Geometry: final body of the model. Coordinates: model frame, mm. A direction names the side the tool comes from. Round coordinates to 2 decimals unless told otherwise and drop trailing zeros. Loops run counter-clockwise (first coordinate to the right, second up) from the corner with the lowest first, then second, coordinate; pieces in that order, holes last. Notation, with made-up numbers: (85.5, 4) - (100.5, 4) arc R18 ccw to (100.5, 33) - close; hole circle Ø2 at (-11.75, -17.75). An arc over 180 degrees is marked (long way). Return JSON: item names as keys, results as strings. Group by question number.
1. Section D-D on y = -36.5. Return loops of the section in (x, z) (3 decimals).
2. Set-up query: faces 5 (the face through (4, -6.858, 33)), 6 (the face through (45.8, -0.2, 38.1)), 7 (the face through (37.434, -9.855, 55.828)), 8 (the face through (41.275, 0, 4)). Return all of +Z, -Z, +X, -X, +Y, -Y with unobstructed straight access to the full face (end or side cutting, diameter ignored); none if empty.
3. Section A-A on y = -24.5. Return loops of the section in (x, z) (3 decimals).
4. Section B-B on z = 5. Return loops of the section in (x, y) (3 decimals), and give its area (3 significant figures).
5. Draft query along X for faces 1 (the face through (60, 0, 42.875)), 2 (the face through (56, 14.478, 45)), 3 (the face through (139.48, -0.97, 52.19)), 4 (the face through (61.811, 0, 41)). Return one class per face: +X half, -X half, draft (parallel to the pull), parting line (faces both ways), or undercut.
6. Section C-C on x = 111. Return loops of the section in (y, z) (3 decimals), and give its area (3 significant figures).
7. Material intervals for probe 1 along Z at (x, y) = (81.5, -8.5) (3 decimals); probe 2 along Y at (x, z) = (24, 42); probe 3 along Z at (x, y) = (38, -25.5) (3 decimals), sorted ascending.
8. First-contact query: pin 1 Ø2.5 at (y, z) = (-1.5, 40) entering from -X; pin 2 Ø16 at (x, y) = (108, -3.5) entering from -Z; pin 3 Ø5 at (y, z) = (-2.5, 65.5) entering from -X; pin 4 Ø8 at (x, y) = (61, -5.5) entering from +Z (3 decimals). Flat tips, straight axial feed; report the tip coordinate or a pass-through.
from build123d import *

# Parameters (mm, degrees)
F1_DEPTH = 41.91
F0_W     = 23.9135493911
F0_H     = 19.0500000095
F0_H_2   = 4.7497999905
F0_H_3   = 4.7752
F2_DEPTH = 14.478
F3_DEPTH = 6.858
F5_R     = 15.24
F6_SIZE  = 5.08


with BuildPart() as f1:
    # F0 (on Front) → F1 (new body, symmetric)
    with BuildSketch(Plane.XZ):
        Polygon((22.2249999905, 9.525), (-41.275, 9.525), (-41.275, -9.525), (41.275, -9.525), (41.275, 9.525), align=None)
    extrude(amount=F1_DEPTH, both=True)

    # F0 (on Front) → F2 (join, symmetric)
    with BuildSketch(Plane.XZ):
        with Locations((73.7682253044, 52.4002000047)):
            Rectangle(F0_W, F0_H)
        Polygon((85.725, 66.675), (85.725, 61.9252000095), (85.725, 42.8752), (85.725, 38.1), (112.6114506089, 38.1), (112.6114506089, 66.675), align=None)
        with Locations((73.7682253044, 64.3001000047)):
            Rectangle(F0_W, F0_H_2)
        with Locations((73.7682253044, 40.4876)):
            Rectangle(F0_W, F0_H_3)
        with BuildLine():
            Line((22.2249999905, 27.0002), (22.2249999905, 9.525))
            Line((22.2249999905, 9.525), (41.275, 9.525))
            Line((41.275, 9.525), (41.275, 27.0002))
            ThreePointArc((41.275, 27.0002), (45.9246798487, 38.2255201513), (57.15, 42.8752))
            Line((57.15, 42.8752), (61.8114506089, 42.8752))
            Line((61.8114506089, 42.8752), (61.8114506089, 61.9252000095))
            Line((61.8114506089, 61.9252000095), (57.15, 61.9252000095))
            ThreePointArc((57.15, 61.9252000095), (52.4471910202, 61.6071243557), (47.8300426869, 60.6586910735))
            ThreePointArc((47.8300426869, 60.6586910735), (29.3538209918, 48.1456027677), (22.2249999905, 27.0002))
        make_face()
    extrude(amount=F2_DEPTH, both=True)

    # F0 (on Front) → F3 (join, symmetric)
    with BuildSketch(Plane.XZ):
        with BuildLine():
            add(Edge.make_bspline(
                [(-41.275, 9.525), (-40.409822017, 35.7104353607), (5.303404294, 69.4405809045), (47.8300426869, 60.6586910735)],
                knots=[0, 0, 0, 0, 102.734429453, 102.734429453, 102.734429453, 102.734429453], degree=3))
            Line((-41.275, 9.525), (22.2249999905, 9.525))
            Line((22.2249999905, 9.525), (22.2249999905, 27.0002))
            ThreePointArc((22.2249999905, 27.0002), (29.3538209918, 48.1456027677), (47.8300426869, 60.6586910735))
        make_face()
    extrude(amount=F3_DEPTH, both=True)

    # F0 (on Front) → F4 (revolve)
    with BuildSketch(Plane.XZ):
        Polygon((85.725, 66.675), (85.725, 61.9252000095), (85.725, 42.8752), (85.725, 38.1), (112.6114506089, 38.1), (112.6114506089, 66.675), align=None)
    revolve(axis=Axis((112.6114506089, 0, 52.3875), (0, 0, 1)))

    # F5
    f5_edges = [f1.edges().sort_by_distance(p)[0] for p in [
        (-41.275, -41.91, 0),
        (41.275, -41.91, 0),
        (41.275, 41.91, 0),
        (-41.275, 41.91, 0),
    ]]
    fillet(f5_edges, radius=F5_R)

    # F6
    f6_edges = [f1.edges().sort_by_distance(p)[0] for p in [
        (61.811451, -14.478, 64.3001),
        (61.811451, -14.478, 40.4876),
        (61.811451, 14.478, 64.3001),
        (61.811451, 14.478, 40.4876),
    ]]
    chamfer(f6_edges, length=F6_SIZE)


solid = f1.part
Taken from the geometry:
{
 "1": {"outline": "(-37.681, -9.525) - (37.681, -9.525) - (37.681, 9.525) - (-37.681, 9.525) - close"},
 "2": {"face 5": "+Z, -X, -Y", "face 6": "-Z, +Y, -Y", "face 7": "+Z", "face 8": "-Z, +X, +Y, -Y"},
 "3": {"outline": "(-41.275, -9.525) - (41.275, -9.525) - (41.275, 9.525) - (-41.275, 9.525) - close; (101.538, 38.1) - (123.685, 38.1) - (123.685, 66.675) - (101.538, 66.675) - close"},
 "4": {"outline": "(-41.275, -26.67) arc R15.24 ccw to (-26.035, -41.91) - (26.035, -41.91) arc R15.24 ccw to (41.275, -26.67) - (41.275, 26.67) arc R15.24 ccw to (26.035, 41.91) - (-26.035, 41.91) arc R15.24 ccw to (-41.275, 26.67) - close", "area": "6,720 mm2"},
 "5": {"face 1": "undercut", "face 2": "draft", "face 3": "parting line", "face 4": "undercut"},
 "6": {"outline": "(-26.838, 38.1) - (26.838, 38.1) - (26.838, 66.675) - (-26.838, 66.675) - close", "area": "1,530 mm2"},
 "7": {"probe 1": "38.1 to 66.675", "probe 2": "-6.86 to 6.86", "probe 3": "-9.525 to 9.525"},
 "8": {"pin 1": "x = -24.77", "pin 2": "z = 38.1", "pin 3": "x = 61.81", "pin 4": "z = 66.675"}
}
